The model under review builds one solid part; all positions refer to its coordinate system, in mm. A direction names the side the tool comes from. Round coordinates to 2 decimals unless told otherwise and drop trailing zeros. Write each loop counter-clockwise with the first axis right and the second up, starting at its lowest first coordinate (ties: lowest second). Pieces come first, ordered by that corner, then holes. Notation, with made-up numbers: M 70.5,-25.75 L 101.5,-25.75 A15 ccw 101.5,2.25 Z; hole C 68,10.5 d8. An arc over 180 degrees is marked long. Write item = value, one per line. Start each with the question number.
Item 1: Take a section at B-B, the plane y = 4. Give the boundary of the cut face in (x, z).
Item 2: Tool access review of faces 5 (the flat face through (11, 12, 6)), 6 (the flat face through (63.25, 9.2, 5.4)), 7 (the flat face through (78, 4, 4)): name each direction out of +Z, -Z, +X, -X, +Y, -Y from which nothing blocks a thin tool from reaching the whole face with its end or side.
Item 3: To check wall thickness, follow line 1 along X through (y, z) = (11.5, 3.75); line 2 along X through (y, z) = (1, 7.75). State the ranges of each line that lie inside material, in increasing order.
Item 4: For pin 1 Ø2.5 at (x, z) = (8, 6.5) entering from +Y; pin 2 Ø5 at (x, y) = (82.5, 2) entering from -Z; pin 3 Ø2.5 at (y, z) = (5.5, 5.5) entering from +X; pin 4 Ø1.5 at (y, z) = (12, 6) entering from +X, all flat-tipped, find the tip position at first contact; note any pin that passes through.
Item 5: Take a section at C-C, the plane x = 87. Give the boundary of the cut face in (y, z).
Item 6: The part is to be moulded in two halves that separate along X. For faces 1 (the flat face through (36, 9, 3.5)), 2 (the flat face through (59.75, 6, 6)), 3 (the flat face through (2.25, 6, 6)), 4 (the flat face through (54, 12, 6)), say which applies: +X half, -X half, draft (parallel to the pull), parting line (faces both ways), or undercut.
Item 7: Take a section at D-D, the plane y = 10.5. Give the boundary of the cut face in (x, z), plus the area to 3 significant figures.
Item 8: Take a section at A-A, the plane z = 7. Give the boundary of the cut face in (x, y), plus the area to 3 significant figures.
Autodesk Fusion 360 part; units mm, degrees
sketch "Sketch1" plane through (0, 0, 0) normal (0, 0, 1) x (1, 0, 0)
  line L0 (0, 0) -> (95, 0)
  line L1 (95, 0) -> (95, 14)
  line L2 (95, 14) -> (0, 14)
  line L3 (0, 14) -> (0, 0)
  dimension "d1" = 95
  dimension "d2" = 14
extrude "Extrude1" add sketch "Sketch1" along normal blind 3.5
sketch "Sketch2" plane through (0, 0, 3.5) normal (0, 0, 1) x (-1, 0, 0)
  line L0 (0, -14) -> (0, 0)
  line L1 (0, 0) -> (-95, 0)
  line L2 (-95, 0) -> (-95, -14)
  line L3 (-95, -14) -> (0, -14)
  line L4 (-2.25, 0) -> (-59.75, 0)
  line L5 (-59.75, 0) -> (-59.75, -12)
  line L6 (-59.75, -12) -> (-2.25, -12)
  line L7 (-2.25, -12) -> (-2.25, 0)
  line L8 (-63.25, 0) -> (-92.75, 0)
  line L9 (-92.75, 0) -> (-92.75, -12)
  line L10 (-92.75, -12) -> (-63.25, -12)
  line L11 (-63.25, -12) -> (-63.25, 0)
  dimension "d5" = 57.5
  dimension "d6" = 12
  dimension "d7" = 2.25
  dimension "d8" = 29.5
  dimension "d9" = 12
  dimension "d22" = 2.25
extrude "Extrude6" add sketch "Sketch2" along normal blind 0.5 contours L1 L8 L9 L10 L11
extrude "Extrude7" add sketch "Sketch2" along normal blind 5 contours L1 L4 L5 L6 L7
sketch "Sketch5" plane through (0, 0, 4) normal (0, 0, 1) x (-1, 0, 0)
  line L0 (-63.25, -12) -> (-63.25, 0)
  line L1 (-63.25, 0) -> (-92.75, 0)
  line L2 (-92.75, 0) -> (-92.75, -12)
  line L3 (-92.75, -12) -> (-63.25, -12)
  line L4 (-63.25, -12) -> (-92.75, -12)
  line L5 (-92.75, -12) -> (-92.75, -9)
  line L6 (-92.75, -9) -> (-63.25, -9)
  line L7 (-63.25, -9) -> (-63.25, -12)
  dimension "d27" = 3
extrude "Extrude8" add sketch "Sketch5" along normal blind 4.5 contours L0 L2 L3 L4 L5 L6 L7
sketch "Sketch6" plane through (0, 0, 8.5) normal (0, 0, 1) x (-1, 0, 0)
  line L0 (-2.25, -12) -> (-2.25, 0)
  line L1 (-2.25, 0) -> (-59.75, 0)
  line L2 (-59.75, 0) -> (-59.75, -12)
  line L3 (-59.75, -12) -> (-2.25, -12)
  line L4 (-20, -12) -> (-47.25, -12)
  line L5 (-47.25, -12) -> (-47.25, 0)
  line L6 (-47.25, 0) -> (-20, 0)
  line L7 (-20, 0) -> (-20, -12)
  line L8 (-2.25, -12) -> (-2.25, 0)
  dimension "d30" = 17.75
  dimension "d31" = 27.25
extrude "Extrude9" cut sketch "Sketch6" against normal blind 5 contours L1 L3 L4 L5 L6 L7
fillet "Fillet1" radius 0.5 6 edges at (92.75, 12, 6) (63.25, 12, 6) (47.25, 12, 6) (20, 12, 6) (2.25, 12, 6) (59.75, 12, 6)
Response values:
q1.outline = M 0,0 L 95,0 L 95,3.5 L 92.75,3.5 L 92.75,4 L 63.25,4 L 63.25,3.5 L 59.75,3.5 L 59.75,8.5 L 47.25,8.5 L 47.25,3.5 L 20,3.5 L 20,8.5 L 2.25,8.5 L 2.25,3.5 L 0,3.5 Z
q2.face_5 = +Z, +X, -X, +Y
q2.face_6 = +Z, +Y, -Y
q2.face_7 = +Z, +X, -Y
q3.line_1 = 2.25 to 20, 47.25 to 59.75, 63.25 to 92.75
q3.line_2 = 2.25 to 20, 47.25 to 59.75
q4.pin_1 = 12
q4.pin_2 = 0
q4.pin_3 = 59.75
q4.pin_4 = 92.75
q5.outline = M 0,0 L 14,0 L 14,3.5 L 12,3.5 L 12,8.5 L 9,8.5 L 9,4 L 0,4 Z
q6.face_1 = undercut
q6.face_2 = undercut
q6.face_3 = -X half
q6.face_4 = draft
q7.outline = M 0,0 L 95,0 L 95,3.5 L 92.75,3.5 L 92.75,8.5 L 63.25,8.5 L 63.25,3.5 L 59.75,3.5 L 59.75,8.5 L 47.25,8.5 L 47.25,3.5 L 20,3.5 L 20,8.5 L 2.25,8.5 L 2.25,3.5 L 0,3.5 Z
q7.area = 631 mm2
q8.outline = M 2.25,0 L 20,0 L 20,11.5 A0.5 ccw 19.5,12 L 2.75,12 A0.5 ccw 2.25,11.5 Z; M 47.25,0 L 59.75,0 L 59.75,11.5 A0.5 ccw 59.25,12 L 47.75,12 A0.5 ccw 47.25,11.5 Z; M 63.25,9 L 92.75,9 L 92.75,11.5 A0.5 ccw 92.25,12 L 63.75,12 A0.5 ccw 63.25,11.5 Z
q8.area = 451 mm2
